```python
from build123d import *

# Parameters (mm, degrees)
CHANFREIN1_SIZE         = 1
CHANFREIN2_SIZE         = 0.5
ESQUISSE2_R             = 2.25
ENL_V_MAT_EXTRU_1_DEPTH = 29.478061732


with BuildPart() as part:
    # Esquisse1 → Base-Révolution (revolve)
    with BuildSketch(Plane.XY, mode=Mode.PRIVATE) as base_r_volution_sk:
        Polygon((-3, 0), (-3, 15), (0, 15), (0, 6), (16, 6), (16, 0), align=None)
    revolve(base_r_volution_sk.sketch.rotate(Axis((-27.336707152, 0, 0), (1, 0, 0)), 90), axis=Axis((-27.336707152, 0, 0), (1, 0, 0)))

    # Chanfrein1
    chanfrein1_edges = [part.edges().sort_by_distance(p)[0] for p in [
        (16, 0, -6),
    ]]
    chamfer(chanfrein1_edges, length=CHANFREIN1_SIZE)

    # Chanfrein2
    chanfrein2_edges = [part.edges().sort_by_distance(p)[0] for p in [
        (-3, 0, -15),
        (0, 0, -15),
    ]]
    chamfer(chanfrein2_edges, length=CHANFREIN2_SIZE)

    # Esquisse2 → Enlèv. mat.-Extru.1 (cut, through all)
    with BuildSketch(Plane.ZY.offset(3)):
        with Locations((0, 11)):
            Circle(ESQUISSE2_R)
    extrude(amount=-ENL_V_MAT_EXTRU_1_DEPTH, mode=Mode.SUBTRACT)


solid = part.part
```
The listing builds one solid part. Answer for the finished solid, in the listing's coordinates (mm). A direction names the side the tool comes from. Round coordinates to 2 decimals unless told otherwise and drop trailing zeros. Loops run counter-clockwise (first coordinate to the right, second up) from the corner with the lowest first, then second, coordinate; pieces in that order, holes last. Notation, with made-up numbers: (89, 63.5) - (130, 63.5) arc R7 ccw to (130, 71.5) - close; hole circle Ø6 at (25.25, 59.5). An arc over 180 degrees is marked (long way). Use one line per item in the form item = value. Start each with the question number.
1. The part is cut by section C-C on x = -2. Determine the outline of the cut face in (y, z).
2. The part is cut by section A-A on z = 0. Determine the outline of the cut face in (x, y), then the cut area to 3 significant figures.
3. Consider line 1 (Y direction, x = -2.1, z = 0); line 2 (X direction, y = -5.75, z = 8); line 3 (Y direction, x = 2.25, z = -1.25). Determine where each line is inside the solid, lowest interval first. Write a range as [from, to].
4. Given pin 1 Ø6 at (x, y) = (5.5, -10) entering from +Z; pin 2 Ø1.5 at (x, z) = (-0.5, 8.5) entering from +Y; pin 3 Ø8 at (x, y) = (6.5, 2) entering from -Z; pin 4 Ø8 at (x, y) = (7, 8.5) entering from -Z, each flat-ended and moving along its own axis, determine where each tip first touches the part or whether it passes through.
5. The part is cut by section B-B on y = 0. Determine the outline of the cut face in (x, z).
6. The part is cut by section D-D on x = 8.5. Determine the outline of the cut face in (y, z), then the cut area to 3 significant figures.
7. For a pull along Z with two mould halves and no side action, classify faces 1 (the face through (-1.52, 13.23, -0.29)), 2 (the face through (-1.49, -12.65, 8.06)), 3 (the face through (-3, 0, 0)) as pulls with the +Z half, pulls with the -Z half, needs draft (parallel to the pull), parting line crosses it, or undercut.
8. A tool of negligible diameter and unlimited length cuts with its end or side. For faces 4 (the face through (16, 0, 0)), 5 (the face through (7.605, -1.802, 5.723)), from which of +Z, -Z, +X, -X, +Y, -Y can it reach the whole face along a straight path? Write none if from no direction.
Geometry check:
q1.outline = circle Ø30 at (0, 0); hole circle Ø4.5 at (11, 0)
q2.outline = (-3, -14.5) - (-2.5, -15) - (-0.5, -15) - (0, -14.5) - (0, -6) - (15, -6) - (16, -5) - (16, 5) - (15, 6) - (0, 6) - (0, 8.75) - (-3, 8.75) - close; (-3, 13.25) - (0, 13.25) - (0, 14.5) - (-0.5, 15) - (-2.5, 15) - (-3, 14.5) - close
q2.area = 267 mm^2
q3.line_1 = [-15, 8.75], [13.25, 15]
q3.line_2 = [-3, 0]
q3.line_3 = [-5.87, 5.87]
q4.pin_1 = through
q4.pin_2 = 12.84
q4.pin_3 = -6
q4.pin_4 = -3.97
q5.outline = (-3, -14.5) - (-2.5, -15) - (-0.5, -15) - (0, -14.5) - (0, -6) - (15, -6) - (16, -5) - (16, 5) - (15, 6) - (0, 6) - (0, 14.5) - (-0.5, 15) - (-2.5, 15) - (-3, 14.5) - close
q6.outline = circle Ø12 at (0, 0)
q6.area = 113 mm^2
q7.face_1 = undercut
q7.face_2 = parting line crosses it
q7.face_3 = needs draft
q8.face_4 = +Z, -Z, +X, +Y, -Y
q8.face_5 = +X
